Drawing for the job (mm, zero at the part's lowest x, y, z). Coordinates: 2 decimals unless noted, no trailing zeros. Write each loop counter-clockwise with the first axis right and the second up, starting at its lowest first coordinate (ties: lowest second). Pieces come first, ordered by that corner, then holes. Notation, with made-up numbers: M 79,87.25 L 90,87.25 A17 ccw 90,92.25 Z; hole C 43.5,4.25 d1. An arc over 180 degrees is marked long. Put each result on its own line as item: value. Start each with the question number.
Q1. Cut at A-A (x = 5.25). Write the cut outline in (y, z).
Q2. Drill centre lines: line 1 along X through (y, z) = (2.95, 5.25); line 2 along X through (y, z) = (5, 5.25); line 3 along Z through (x, y) = (3.5, 2). Where is each one in solid material? Low to high.
Q3. Pull direction X, two halves, no side cores. Call the marked faces 1, 2 and 3: pulls with the +X half, pulls with the -X half, needs draft (parallel to the pull), parting line crosses it, or undercut.
Q4. Cut at B-B (z = 5.25). Write the cut outline in (x, y), then the cut area to 3 significant figures.
Q5. Drop flat-ended pins along their axis: pin 1 (1.5 mm diameter, centred on x = 2.5, y = 7.5, fed in from -Z); pin 2 (1.5 mm diameter, centred on y = 6.5, z = 6.5, fed in from -X); pin 3 (4.5 mm diameter, centred on x = 5.25, z = 5.25, fed in from -Y). Give the stop position or say it passes through.
Q6. Cut at C-C (y = 1). Write the cut outline in (x, z).
Q7. Cut at D-D (z = 2.5). Write the cut outline in (x, y), then the cut area to 3 significant figures.
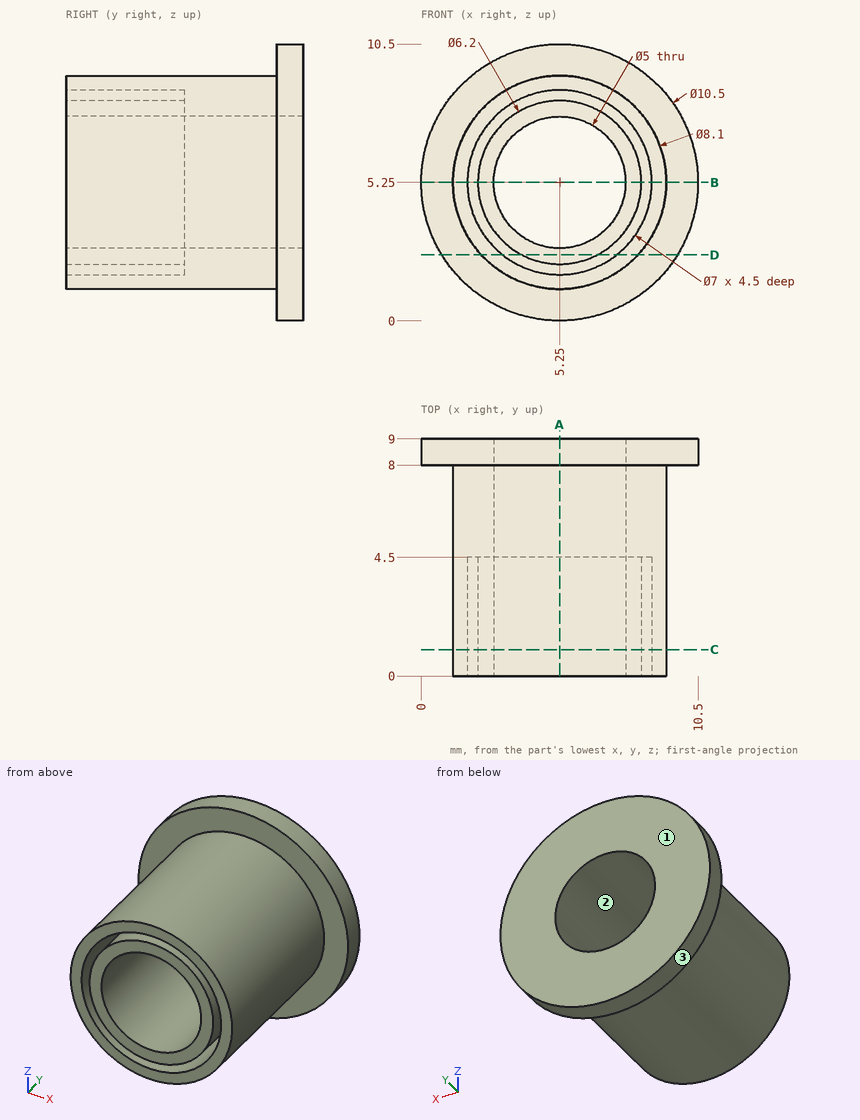
Computed values:
1. outline: M 0,1.2 L 8,1.2 L 8,0 L 9,0 L 9,2.75 L 0,2.75 L 0,2.15 L 4.5,2.15 L 4.5,1.75 L 0,1.75 Z; M 0,7.75 L 9,7.75 L 9,10.5 L 8,10.5 L 8,9.3 L 0,9.3 L 0,8.75 L 4.5,8.75 L 4.5,8.35 L 0,8.35 Z
2. line 1: 1.2 to 1.75, 2.15 to 2.75, 7.75 to 8.35, 8.75 to 9.3
2. line 2: 1.2 to 2.75, 7.75 to 9.3
2. line 3: 1.6 to 2.22, 2.69 to 3.46, 7.04 to 7.81, 8.28 to 8.9
3. face 1: needs draft
3. face 2: undercut
3. face 3: parting line crosses it
4. outline: M 0,8 L 1.2,8 L 1.2,0 L 1.75,0 L 1.75,4.5 L 2.15,4.5 L 2.15,0 L 2.75,0 L 2.75,9 L 0,9 Z; M 7.75,0 L 8.35,0 L 8.35,4.5 L 8.75,4.5 L 8.75,0 L 9.3,0 L 9.3,8 L 10.5,8 L 10.5,9 L 7.75,9 Z
4. area: 26.7 mm2
5. pin 1: z = 0.48
5. pin 2: x = 1.23
5. pin 3: through
6. outline: C 5.25,5.25 d8.1; C 5.25,5.25 d6.2; hole C 5.25,5.25 d7; hole C 5.25,5.25 d5
7. outline: M 0.78,8 L 2.28,8 L 2.28,0 L 3.08,0 L 3.08,4.5 L 3.82,4.5 L 3.82,0 L 6.68,0 L 6.68,4.5 L 7.42,4.5 L 7.42,0 L 8.22,0 L 8.22,8 L 9.72,8 L 9.72,9 L 0.78,9 Z
7. area: 49.9 mm2
